```python
from build123d import *

# Parameters (mm, degrees)
SKETCH1_W           = 419.1
SKETCH1_H           = 142.18412
BOSS_EXTRUDE1_DEPTH = 88.9
SKETCH2_R           = 119.38
CUT_EXTRUDE1_DEPTH  = 83.4009
SKETCH7_W           = 194.780719179
SKETCH7_H           = 43.63974
SKETCH7_H_2         = 53.35016
CUT_EXTRUDE2_DEPTH  = 452.402640644
SKETCH3_R           = 24.99995
CUT_EXTRUDE3_DEPTH  = 15.24
SKETCH4_R           = 40.25011
CUT_EXTRUDE4_DEPTH  = 10
SKETCH5_R           = 27.50058
CUT_EXTRUDE5_DEPTH  = 2.54
SKETCH8_W           = 419.1
SKETCH8_H           = 88.9
CUT_EXTRUDE6_DEPTH  = 7.85114
SKETCH9_W           = 419.1
SKETCH9_H           = 88.9
CUT_EXTRUDE7_DEPTH  = 11.94308
SKETCH10_W          = 219.202
SKETCH10_H          = 88.9
CUT_EXTRUDE8_DEPTH  = 30.48
SKETCH12_W          = 121.533574186
SKETCH12_H          = 91.9099
BOSS_EXTRUDE2_DEPTH = 25.4
SKETCH14_W          = 55.647095764
SKETCH14_H          = 91.9099
BOSS_EXTRUDE3_DEPTH = 12.7
SKETCH17_R          = 12.827
CUT_EXTRUDE10_DEPTH = 446.564033133


with BuildPart() as part:
    # Sketch1 → Boss-Extrude1 (new body)
    with BuildSketch(Plane(origin=(0, 0, 0), x_dir=(1, 0, 0), z_dir=(0, 1, 0))):
        with Locations((209.55, 71.09206)):
            Rectangle(SKETCH1_W, SKETCH1_H)
    extrude(amount=BOSS_EXTRUDE1_DEPTH)

    # Sketch2 → Cut-Extrude1 (cut)
    with BuildSketch(Plane(origin=(0, 0, -131.63296), x_dir=(-1, 0, 0), z_dir=(0, 0, -1))):
        with Locations((-116.7166499, 150.061217688)):
            Circle(SKETCH2_R)
    extrude(amount=-CUT_EXTRUDE1_DEPTH, mode=Mode.SUBTRACT)

    # Sketch7 → Cut-Extrude2 (cut, through all)
    with BuildSketch(Plane(origin=(0, 88.9, 0), x_dir=(1, 0, 0), z_dir=(0, 1, 0))):
        with Locations((321.709640411, 97.27311)):
            Rectangle(SKETCH7_W, SKETCH7_H)
        with Locations((321.709640411, 41.15816)):
            Rectangle(SKETCH7_W, SKETCH7_H_2)
    extrude(amount=-CUT_EXTRUDE2_DEPTH, mode=Mode.SUBTRACT)

    # Sketch3 → Cut-Extrude3 (cut)
    with BuildSketch(Plane(origin=(0, 0, -134.33298), x_dir=(-1, 0, 0), z_dir=(0, 0, -1))):
        with Locations((-278.649352085, 104.852009966)):
            Circle(SKETCH3_R)
    extrude(amount=-CUT_EXTRUDE3_DEPTH, mode=Mode.SUBTRACT)

    # Sketch4 → Cut-Extrude4 (cut)
    with BuildSketch(Plane(origin=(0, 0, -67.83324), x_dir=(-1, 0, 0), z_dir=(0, 0, -1))):
        with Locations((-278.649352085, 104.852009966)):
            Circle(SKETCH4_R)
    extrude(amount=CUT_EXTRUDE4_DEPTH, mode=Mode.SUBTRACT)

    # Sketch5 → Cut-Extrude5 (cut)
    with BuildSketch(Plane(origin=(0, 0, -14.48308), x_dir=(-1, 0, 0), z_dir=(0, 0, -1))):
        with Locations((-278.649352085, 104.852009966)):
            Circle(SKETCH5_R)
    extrude(amount=-CUT_EXTRUDE5_DEPTH, mode=Mode.SUBTRACT)

    # Sketch8 → Cut-Extrude6 (cut)
    with BuildSketch(Plane(origin=(0, 0, -142.18412), x_dir=(-1, 0, 0), z_dir=(0, 0, -1))):
        with Locations((-209.55, 44.45)):
            Rectangle(SKETCH8_W, SKETCH8_H)
    extrude(amount=-CUT_EXTRUDE6_DEPTH, mode=Mode.SUBTRACT)

    # Sketch9 → Cut-Extrude7 (cut)
    with BuildSketch(Plane.XY):
        with Locations((209.55, 44.45)):
            Rectangle(SKETCH9_W, SKETCH9_H)
    extrude(amount=-CUT_EXTRUDE7_DEPTH, mode=Mode.SUBTRACT)

    # Sketch10 → Cut-Extrude8 (cut)
    with BuildSketch(Plane.XY.offset(-11.94308)):
        with Locations((109.601, 44.45)):
            Rectangle(SKETCH10_W, SKETCH10_H)
    extrude(amount=-CUT_EXTRUDE8_DEPTH, mode=Mode.SUBTRACT)

    # Sketch12 → Boss-Extrude2 (add)
    with BuildSketch(Plane.XZ):
        with Locations((-60.766787093, -88.37803)):
            Rectangle(SKETCH12_W, SKETCH12_H)
    extrude(amount=-BOSS_EXTRUDE2_DEPTH)

    # Sketch14 → Boss-Extrude3 (add)
    with BuildSketch(Plane.XZ):
        with Locations((-93.710026304, -88.37803)):
            Rectangle(SKETCH14_W, SKETCH14_H)
    extrude(amount=BOSS_EXTRUDE3_DEPTH)

    # Sketch17 → Cut-Extrude10 (cut, through all)
    with BuildSketch(Plane(origin=(0, 0, -134.33298), x_dir=(-1, 0, 0), z_dir=(0, 0, -1))):
        with Locations((-384.735935495, 0.531880938)):
            Circle(SKETCH17_R)
        with Locations((94.798916194, -17.274045482)):
            Circle(SKETCH17_R)
        with BuildLine():
            Line((-169.736021607, 19.31637742), (-169.736021607, 0))
            Line((-169.736021607, 0), (-144.082021607, 0))
            Line((-144.082021607, 0), (-144.082021607, 19.31637742))
            ThreePointArc((-144.082021607, 19.31637742), (-156.909021607, 32.14337742), (-169.736021607, 19.31637742))
        make_face()
    extrude(amount=-CUT_EXTRUDE10_DEPTH, mode=Mode.SUBTRACT)


solid = part.part
```
Design review of the part built by this model. Coordinates are the model's own, in mm. A direction names the side the tool comes from. Coordinates: 2 decimals unless noted, no trailing zeros. Order: outer loops, then holes, each group sorted by start corner. A loop starts at its lowest first (then second) coordinate and runs counter-clockwise, first axis right, second up.
1) For faces 1 (the flat face through (144.082, 10, -89)), 2 (the flat face through (224.319, 45, -97)), 3 (the flat face through (-62, 25.4, -88)), 4 (the flat face through (38, 0, -88)), 5 (the flat face through (219.202, 44, -27)), list the 3-axis set-ups (+Z, -Z, +X, -X, +Y, -Y) from which the entire face can be reached by the end or side of a thin tool; tool diameter is ignored.
2) Wall thickness on line 1 along Z through (x, y) = (283, 40.5); line 2 along X through (y, z) = (1.5, -62); line 3 along X through (y, z) = (3, -20): over which ranges is each line inside the solid? List them lowest first.
3) Take a section at D-D, the plane x = -26.5. Give the boundary of the cut face in (y, z), and give its area (3 significant figures).
4) Mouldability with a two-part tool opening along Z and no side actions: class faces 6 (the cylindrical face through (156.63, 32.14, -89.02)), 7 (the flat face through (118, 67, -48.232)) as +Z half, -Z half, draft (parallel to the pull), parting line (faces both ways), or undercut.
5) Take a section at B-B, the plane y = 49.5. Give the boundary of the cut face in (x, z), and give its area (3 significant figures).
6) Take a section at C-C, the plane z = -113.5. Give the boundary of the cut face in (x, y).
7) Clearance check with flat-ended pins moving along their axes: pin 1 (3 mm diameter, centred on x = 406.5, z = -13.5, fed in from -Y); pin 2 (22 mm diameter, centred on y = 51, z = -104, fed in from +X); pin 3 (8 mm diameter, centred on x = 88, y = 22, fed in from +Z). State where each tip first meets the part, or that it passes through.
8) Take a section at A-A, the plane x = 348. Give the boundary of the cut face in (y, z), and give its area (3 significant figures).
Returned:
1. face 1: +Z, -Z, -Y
1. face 2: +X, +Y, -Y
1. face 3: +Z, -Z, -X, +Y
1. face 4: +Z, -Z, +X, -Y
1. face 5: +Z, -X, +Y, -Y
2. line 1: z = -134.33 to -119.09, -75.45 to -67.83, -14.48 to -11.94
2. line 2: x = -121.53 to 144.08, 169.74 to 224.32
2. line 3: x = 219.2 to 224.32
3. outline: (0, -134.33) - (25.4, -134.33) - (25.4, -42.42) - (0, -42.42) - close
3. area: 2,330 mm2
4. face 6: draft
4. face 7: undercut
5. outline: (0, -134.33) - (419.1, -134.33) - (419.1, -119.09) - (224.32, -119.09) - (224.32, -75.45) - (419.1, -75.45) - (419.1, -67.83) - (224.32, -67.83) - (224.32, -14.48) - (419.1, -14.48) - (419.1, -11.94) - (219.2, -11.94) - (219.2, -42.42) - (0, -42.42) - close; hole (52.38, -131.63) - (181.05, -131.63) - (181.05, -48.23) - (52.38, -48.23) - close
5. area: 15,000 mm2
6. outline: (-121.53, -12.7) - (-106.78, -12.7) arc R12.83 cw to (-82.82, -12.7) - (-65.89, -12.7) - (-65.89, 0) - (144.08, 0) - (144.08, 19.32) arc R12.83 cw to (169.74, 19.32) - (169.74, 0) - (224.32, 0) - (224.32, 88.9) - (219.24, 88.9) arc R119.38 cw to (14.19, 88.9) - (0, 88.9) - (0, 25.4) - (-121.53, 25.4) - close
7. pin 1: stops at y = 0
7. pin 2: stops at x = 224.32
7. pin 3: stops at z = -42.42
8. outline: (0, -134.33) - (88.9, -134.33) - (88.9, -119.09) - (0, -119.09) - close; (0, -75.45) - (88.9, -75.45) - (88.9, -67.83) - (0, -67.83) - close; (0, -14.48) - (88.9, -14.48) - (88.9, -11.94) - (0, -11.94) - close
8. area: 2,260 mm2
